Input: part model. Units: mm. Frame: model coordinates. A direction names the side the tool comes from. Give positions to 0.01 mm unless a question says otherwise; leave off trailing zeros. Order: outer loops, then holes, each group sorted by start corner. A loop starts at its lowest first (then second) coordinate and runs counter-clockwise, first axis right, second up. Notation, with made-up numbers: (-29.75, -29.75) - (12.25, -29.75) arc R22 ccw to (12.25, 6.25) - close; hole circle Ø5 at (51.5, 17.5). An arc over 180 degrees is marked (long way). Answer in a Markdown table with one row per item. Add a question column.
from build123d import *

# Parameters (mm, degrees)
BOSS_EXTRUDE1_DEPTH = 6
SKETCH4_R           = 5
CUT_EXTRUDE2_DEPTH  = 262.076617107
CUT_EXTRUDE5_DEPTH  = 262.076617107
FILLET5_R           = 5
FILLET6_R           = 5
SKETCH9_R           = 5
SKETCH9_W           = 55
SKETCH9_H           = 39.899020921
CUT_EXTRUDE6_DEPTH  = 262.076617107


with BuildPart() as part:
    # Sketch1 → Boss-Extrude1 (new body)
    with BuildSketch(Plane.XY):
        with BuildLine():
            Line((-250, -55), (-250, 3.178280867))
            Line((-250, 3.178280867), (-250, 55))
            ThreePointArc((-250, 55), (-244.142135624, 69.142135624), (-230, 75))
            Line((-230, 75), (-220, 75))
            Line((-220, 75), (-164.330865428, 75))
            Line((-164.330865428, 75), (-60, 75))
            ThreePointArc((-60, 75), (-52.928932188, 72.071067812), (-50, 65))
            Line((-50, 65), (-50, 20))
            ThreePointArc((-50, 20), (-48.100925873, 14.1369803), (-43.125, 10.500822404))
            ThreePointArc((-43.125, 10.500822404), (-39.437786703, 8.32242004), (-37, 4.801315846))
            ThreePointArc((-37, 4.801315846), (-22.271648276, -13.226099426), (0, -20))
            Line((0, -20), (0, -40))
            Line((0, -40), (0, -65))
            Line((0, -65), (0, -75))
            Line((0, -75), (-230, -75))
            ThreePointArc((-230, -75), (-244.142135624, -69.142135624), (-250, -55))
        make_face()
    boss_extrude1 = extrude(amount=BOSS_EXTRUDE1_DEPTH)

    # Mirror1: Boss-Extrude1 across plane
    add(boss_extrude1.mirror(Plane(origin=(0, -20, 6), x_dir=(0, 0, 1), z_dir=(-1, 0, 0))))

    # Sketch4 → Cut-Extrude2 (cut, through all)
    with BuildSketch(Plane.XY.offset(6)):
        with Locations((-200, -55)):
            Circle(SKETCH4_R)
        with Locations((-100, -55)):
            Circle(SKETCH4_R)
        with BuildLine():
            Line((-70, 25.100979079), (-70, -54.899020921))
            ThreePointArc((-70, -54.899020921), (-72.928932188, -61.970088733), (-80, -64.899020921))
            Line((-80, -64.899020921), (-90, -64.899020921))
            Line((-90, -64.899020921), (-90, -55))
            ThreePointArc((-90, -55), (-100, -45), (-110, -55))
            Line((-110, -55), (-110, -65))
            Line((-110, -65), (-190, -65))
            Line((-190, -65), (-190, -55))
            ThreePointArc((-190, -55), (-200, -45), (-210, -55))
            Line((-210, -55), (-210, -65))
            Line((-210, -65), (-230, -65))
            ThreePointArc((-230, -65), (-237.071067812, -62.071067812), (-240, -55))
            Line((-240, -55), (-240, 25.100979079))
            ThreePointArc((-240, 25.100979079), (-237.071067812, 32.17204689), (-230, 35.100979079))
            Line((-230, 35.100979079), (-140, 35.100979079))
            Line((-140, 35.100979079), (-110, 35.100979079))
            Line((-110, 35.100979079), (-80, 35.100979079))
            ThreePointArc((-80, 35.100979079), (-72.928932188, 32.17204689), (-70, 25.100979079))
        make_face()
    cut_extrude2 = extrude(amount=-CUT_EXTRUDE2_DEPTH, mode=Mode.SUBTRACT)

    # Mirror2: Cut-Extrude2 across plane
    add(cut_extrude2.mirror(Plane(origin=(0, 0, 0), x_dir=(0, 0, 1), z_dir=(1, 0, 0))), mode=Mode.SUBTRACT)

    # Sketch8 → Cut-Extrude5 (cut, through all)
    with BuildSketch(Plane.XY.offset(6)):
        with BuildLine():
            Line((-60, 0), (-60, -64.899020921))
            Line((-60, -64.899020921), (60, -64.899020921))
            Line((60, -64.899020921), (60, 0))
            ThreePointArc((60, 0), (57.236067977, 4.472135955), (52, 4))
            ThreePointArc((52, 4), (49.247332505, 2.266223145), (46.25, 1.001644808))
            ThreePointArc((46.25, 1.001644808), (0, -30), (-46.25, 1.001644808))
            ThreePointArc((-46.25, 1.001644808), (-49.247332505, 2.266223145), (-52, 4))
            ThreePointArc((-52, 4), (-57.236067977, 4.472135955), (-60, 0))
        make_face()
    extrude(amount=-CUT_EXTRUDE5_DEPTH, mode=Mode.SUBTRACT)

    # Fillet5
    fillet5_edges = [part.edges().sort_by_distance(p)[0] for p in [
        (-60, -64.899020921, 3),
    ]]
    fillet(fillet5_edges, radius=FILLET5_R)

    # Fillet6
    fillet6_edges = [part.edges().sort_by_distance(p)[0] for p in [
        (60, -64.899020921, 3),
    ]]
    fillet(fillet6_edges, radius=FILLET6_R)

    # Sketch9 → Cut-Extrude6 (cut, through all)
    with BuildSketch(Plane(origin=(0, 0, 0), x_dir=(-1, 0, 0), z_dir=(0, 0, -1))):
        with Locations((-200, 55)):
            Circle(SKETCH9_R)
        with Locations((-110, 55)):
            Circle(SKETCH9_R)
        with Locations((80, 55)):
            Circle(SKETCH9_R)
        with Locations((235, 55)):
            Circle(SKETCH9_R)
        with Locations((192.5, 55.05048954)):
            Rectangle(SKETCH9_W, SKETCH9_H)
    extrude(amount=-CUT_EXTRUDE6_DEPTH, mode=Mode.SUBTRACT)


solid = part.part
Q1. Line query: probe 1 along Y at (x, z) = (100, 3.9); probe 2 along X at (y, z) = (43, 1.2); probe 3 along Y at (x, z) = (-80, 2.95). Output: solid intervals per line, ascending.
Q2. Access query for faces 4 (the cylindrical face through (53.01, 72.15, 2.96)), 5 (the cylindrical face through (-236.99, -62.15, 3.04)), 6 (the cylindrical face through (244.297, 68.986, 2.958)). Directions: +Z, -Z, +X, -X, +Y, -Y. A direction counts if a zero-diameter tool reaches every point of the face in a straight line with its end or side. Return the directions, or none.
Q3. Section B-B, the plane x = -235. Return loops of the section in (y, z).
Q4. Section C-C, the plane z = 3.85. State how many separate pieces and enclosed holes the cut face has, then the cut area to 3 significant figures.
Q5. Pull-direction query (Y, two-part tool) for faces 1 (the cylindrical face through (-243.986, -69.297, 2.958)), 2 (the cylindrical face through (-53.01, 72.15, 2.96)), 3 (the cylindrical face through (237.15, 32.09, 3.04)); classes: +Y half, -Y half, draft (parallel to the pull), parting line (faces both ways), or undercut.
Q6. Section A-A, the plane x = -139.5. Return loops of the section in (y, z).
Q7. Contact query for flat-ended pins moving along their axis: P1, Ø3, axis at y = -57.5, z = 2.5, coming from the -X side (3 decimals); P2, Ø1.8, axis at y = 64, z = 4.5, coming from the -X side; P3, Ø1.8, axis at y = -62, z = 2, coming from the +X side; P4, Ø9, axis at x = 200, y = 55, coming from the -Z side. Output: stop coordinate, or through.
Computed:
| question | item | result |
|---|---|---|
| 1 | probe 1 | y = -75 to -60, -50 to -45, 35.1 to 75 |
| 1 | probe 2 | x = -250 to -220, -165 to -50, 50 to 250 |
| 1 | probe 3 | y = -75 to -64.9, 35.1 to 50, 60 to 75 |
| 2 | face 4 | +Z, -Z, +Y |
| 2 | face 5 | +Z, -Z |
| 2 | face 6 | +Z, -Z, +X, +Y |
| 3 | outline | (-74.36, 0) - (-63.66, 0) - (-63.66, 6) - (-74.36, 6) - close; (33.76, 0) - (50, 0) - (50, 6) - (33.76, 6) - close; (60, 0) - (74.36, 0) - (74.36, 6) - (60, 6) - close |
| 4 | separate pieces | 1 |
| 4 | enclosed holes | 10 |
| 4 | area | 25,300 mm^2 |
| 5 | face 1 | -Y half |
| 5 | face 2 | +Y half |
| 5 | face 3 | undercut |
| 6 | outline | (-75, 0) - (-65, 0) - (-65, 6) - (-75, 6) - close; (35.1, 0) - (75, 0) - (75, 6) - (35.1, 6) - close |
| 7 | P1 | stops at x = -249.975 |
| 7 | P2 | stops at x = -248.29 |
| 7 | P3 | stops at x = 249.05 |
| 7 | P4 | passes through |
